from build123d import *

# Parameters (mm, degrees)
F1_DEPTH     = 76.2
F2_T1_DEPTH  = 175.4963381321
F2_T3_DEPTH  = 175.4963381321
F2_T5_DEPTH  = 175.4963381321
F2_T7_DEPTH  = 175.4963381321
F2_T9_DEPTH  = 175.4963381321
F2_T11_DEPTH = 175.4963381321
F2_T13_DEPTH = 175.4963381321


# Not quite as in the source:
# - a fillet or chamfer that OpenCascade refuses, or shapes differently, is made with other operations: its cross-section is extruded or revolved along the edge and cut away or added


with BuildPart() as f1:
    # F0 (on Top) → F1 (new body, symmetric)
    with BuildSketch(Plane.XY):
        Polygon((0, 0), (0, 55.7593321666), (-0.2656214809, 55.8856970104), (-43.8588096269, 34.6364909196), align=None)
        Polygon((0, 0), (43.5275850579, 35.051833392), (0, 55.7593321666), align=None)
        Polygon((51.7034059885, 0), (43.5275850579, 35.051833392), (0, 0), align=None)
        Polygon((24.487211867, -50.2360243261), (54.5436322472, -12.1767756978), (0, 0), align=None)
        Polygon((0, -50.3524106258), (0, 0), (-24.0085784972, -50.4665220087), align=None)
        Polygon((24.487211867, -50.2360243261), (0, 0), (0, -50.3524106258), align=None)
        Polygon((-24.0085784972, -50.4665220087), (0, 0), (-54.4254195672, -12.6946992894), align=None)
        Polygon((-51.5913489447, 0), (0, 0), (-43.8588096269, 34.6364909196), align=None)
        Polygon((-54.4254195672, -12.6946992894), (0, 0), (-51.5913489447, 0), align=None)
        Polygon((0, 0), (54.5436322472, -12.1767756978), (51.7034059885, 0), align=None)
    extrude(amount=F1_DEPTH, both=True)

    # F2: fillet of radius 25.4 on 14 edges, made by hand

    # F2_s2 → F2_t1 (cut)
    with BuildSketch(Plane(origin=(78.8765212158, 38.447829267, 0), x_dir=(0, 0, 1), z_dir=(-0.8988964904, -0.4381610429, 0))):
        with BuildLine():
            ThreePointArc((-50.8, 50.3518418934), (-68.7605122421, 42.9123541355), (-76.2, 24.9518418934))
            Line((-76.2, 24.9518418934), (-76.2, 50.3518418934))
            Line((-76.2, 50.3518418934), (-50.8, 50.3518418934))
        make_face()
        with BuildLine():
            ThreePointArc((50.8, 50.3518418934), (68.7605122421, 42.9123541355), (76.2, 24.9518418934))
            Line((76.2, 24.9518418934), (76.2, 50.3518418934))
            Line((76.2, 50.3518418934), (50.8, 50.3518418934))
        make_face()
    extrude(amount=F2_T1_DEPTH, mode=Mode.SUBTRACT)

    # F2_s4 → F2_t3 (cut)
    with BuildSketch(Plane(origin=(19.1189832306, 85.6399769656, 0), x_dir=(0, 0, 1), z_dir=(-0.217884697, -0.9759745175, 0))):
        with BuildLine():
            ThreePointArc((-50.8, 50.3518418934), (-68.7605122421, 42.9123541355), (-76.2, 24.9518418934))
            Line((-76.2, 24.9518418934), (-76.2, 50.3518418934))
            Line((-76.2, 50.3518418934), (-50.8, 50.3518418934))
        make_face()
        with BuildLine():
            ThreePointArc((76.2, 24.9518418934), (68.7605122421, 42.9123541355), (50.8, 50.3518418934))
            Line((50.8, 50.3518418934), (76.2, 50.3518418934))
            Line((76.2, 50.3518418934), (76.2, 24.9518418934))
        make_face()
    extrude(amount=F2_T3_DEPTH, mode=Mode.SUBTRACT)

    # F2_s6 → F2_t5 (cut)
    with BuildSketch(Plane(origin=(-55.0355390834, 68.343475272, 0), x_dir=(0, 0, 1), z_dir=(0.6271987173, -0.7788592742, 0))):
        with BuildLine():
            ThreePointArc((-50.8, 50.3518418934), (-68.7605122421, 42.9123541355), (-76.2, 24.9518418934))
            Line((-76.2, 24.9518418934), (-76.2, 50.3518418934))
            Line((-76.2, 50.3518418934), (-50.8, 50.3518418934))
        make_face()
        with BuildLine():
            ThreePointArc((50.8, 50.3518418934), (68.7605122421, 42.9123541355), (76.2, 24.9518418934))
            Line((76.2, 24.9518418934), (76.2, 50.3518418934))
            Line((76.2, 50.3518418934), (50.8, 50.3518418934))
        make_face()
    extrude(amount=F2_T5_DEPTH, mode=Mode.SUBTRACT)

    # F2_s8 → F2_t7 (cut)
    with BuildSketch(Plane(origin=(-87.7471779472, -0.4170572543, 0), x_dir=(0, 0, 1), z_dir=(0.999988705, 0.0047528884, 0))):
        with BuildLine():
            ThreePointArc((-50.8, 50.3518418934), (-68.7605122421, 42.9123541355), (-76.2, 24.9518418934))
            Line((-76.2, 24.9518418934), (-76.2, 50.3518418934))
            Line((-76.2, 50.3518418934), (-50.8, 50.3518418934))
        make_face()
        with BuildLine():
            ThreePointArc((50.8, 50.3518418934), (68.7605122421, 42.9123541355), (76.2, 24.9518418934))
            Line((76.2, 24.9518418934), (76.2, 50.3518418934))
            Line((76.2, 50.3518418934), (50.8, 50.3518418934))
        make_face()
    extrude(amount=F2_T7_DEPTH, mode=Mode.SUBTRACT)

    # F2_s10 → F2_t9 (cut)
    with BuildSketch(Plane(origin=(-54.3834021005, -68.8635371617, 0), x_dir=(0, 0, 1), z_dir=(0.6197668017, 0.7847860291, 0))):
        with BuildLine():
            ThreePointArc((-50.8, 50.3518418934), (-68.7605122421, 42.9123541355), (-76.2, 24.9518418934))
            Line((-76.2, 24.9518418934), (-76.2, 50.3518418934))
            Line((-76.2, 50.3518418934), (-50.8, 50.3518418934))
        make_face()
        with BuildLine():
            ThreePointArc((50.8, 50.3518418934), (68.7605122421, 42.9123541355), (76.2, 24.9518418934))
            Line((76.2, 24.9518418934), (76.2, 50.3518418934))
            Line((76.2, 50.3518418934), (50.8, 50.3518418934))
        make_face()
    extrude(amount=F2_T9_DEPTH, mode=Mode.SUBTRACT)

    # F2_s12 → F2_t11 (cut)
    with BuildSketch(Plane(origin=(19.932184747, -85.4543690261, 0), x_dir=(0, 0, 1), z_dir=(-0.2271521441, 0.9738592832, 0))):
        with BuildLine():
            ThreePointArc((-50.8, 50.3518418934), (-68.7605122421, 42.9123541355), (-76.2, 24.9518418934))
            Line((-76.2, 24.9518418934), (-76.2, 50.3518418934))
            Line((-76.2, 50.3518418934), (-50.8, 50.3518418934))
        make_face()
        with BuildLine():
            ThreePointArc((50.8, 50.3518418934), (68.7605122421, 42.9123541355), (76.2, 24.9518418934))
            Line((76.2, 24.9518418934), (76.2, 50.3518418934))
            Line((76.2, 50.3518418934), (50.8, 50.3518418934))
        make_face()
    extrude(amount=F2_T11_DEPTH, mode=Mode.SUBTRACT)

    # F2_s14 → F2_t13 (cut)
    with BuildSketch(Plane(origin=(79.2384299376, -37.6963180625, 0), x_dir=(0, 0, 1), z_dir=(-0.9030208924, 0.4295966339, 0))):
        with BuildLine():
            ThreePointArc((-50.8, 50.3518418934), (-68.7605122421, 42.9123541355), (-76.2, 24.9518418934))
            Line((-76.2, 24.9518418934), (-76.2, 50.3518418934))
            Line((-76.2, 50.3518418934), (-50.8, 50.3518418934))
        make_face()
        with BuildLine():
            ThreePointArc((50.8, 50.3518418934), (68.7605122421, 42.9123541355), (76.2, 24.9518418934))
            Line((76.2, 24.9518418934), (76.2, 50.3518418934))
            Line((76.2, 50.3518418934), (50.8, 50.3518418934))
        make_face()
    extrude(amount=F2_T13_DEPTH, mode=Mode.SUBTRACT)


solid = f1.part
Geometry check sheet. Reference: the model listing, model coordinates, mm. A direction names the side the tool comes from. Coordinates: 2 decimals unless noted, no trailing zeros. Order: outer loops, then holes, each group sorted by start corner. A loop starts at its lowest first (then second) coordinate and runs counter-clockwise, first axis right, second up. Notation, with made-up numbers: (-13.75, -7) - (42.25, -7) arc R30 ccw to (42.25, 32) - close; hole circle Ø6 at (32.25, 70). An arc over 180 degrees is marked (long way). Answer in a Markdown table with one row per item. Add a question column.
1) Cross-section at C-C, the plane z = -60.5. Record the cut outline in (x, y), then the cut area to 3 significant figures.
2) Gauge pin test, flat ends, axial feed: P1, Ø5, axis at y = 20, z = -56, coming from the -X side; P2, Ø1, axis at y = -0.5, z = 39.5, coming from the -X side; P3, Ø3, axis at y = -4.5, z = -5, coming from the -X side. Record the tip position at first contact, or that the pin passes through.
3) Material ranges on line 1 along Y through (x, z) = (-11.5, -3.5); line 2 along X through (y, z) = (-13, -68); line 3 along X through (y, z) = (-23.5, -57), recorded low to high. Write a range as [from, to].
4) Set-up check for faces 1 (the cylindrical face through (-44.74, 10.34, -65.14)), 2 (the cylindrical face through (-0.12, -45.92, 65.14)), 3 (the cylindrical face through (-0.12, -45.92, -65.14)): record each of +Z, -Z, +X, -X, +Y, -Y from which the full face is reachable in a straight line by a thin tool's end or side.
5) Cross-section at B-B, the plane z = 62. Record the cut outline in (x, y).
6) Cross-section at A-A, the plane z = 14. Record the cut outline in (x, y).
Check result:
| question | item | result |
|---|---|---|
| 1 | outline | (-52.34, -12.21) - (-23.09, -48.54) - (23.55, -48.32) - (52.46, -11.71) - (41.86, 33.71) - (-0.26, 53.75) - (-42.18, 33.31) - close |
| 1 | area | 7,910 mm² |
| 2 | P1 | stops at x = -47.3 |
| 2 | P2 | stops at x = -51.81 |
| 2 | P3 | stops at x = -52.93 |
| 3 | line 1 | y = [-50.41, 50.41] |
| 3 | line 2 | x = [-45.56, 45.34] |
| 3 | line 3 | x = [-44.74, 44.62] |
| 4 | face 1 | -Z, -X, +Y |
| 4 | face 2 | +Z, +X, -Y |
| 4 | face 3 | -Z, +X, -Y |
| 5 | outline | (-51.61, -12.04) - (-22.77, -47.86) - (23.22, -47.64) - (51.72, -11.55) - (41.28, 33.24) - (-0.25, 53) - (-41.59, 32.85) - close |
| 6 | outline | (-54.43, -12.69) - (-24.01, -50.47) - (24.49, -50.24) - (54.54, -12.18) - (43.53, 35.05) - (-0.27, 55.89) - (-43.86, 34.64) - close |
